```python
from build123d import *

# Parameters (mm, degrees)
REVOLUTION007_ANGLE     = 180
SKETCH064_W             = 14
SKETCH064_H             = 6
PAD026_DEPTH            = 10
SKETCH063_R             = 1.7
POCKET007_DEPTH         = 38.901
POCKET008_DEPTH         = 28.901
BODY015_PLACEMENT_ANGLE = 180


with BuildPart() as part:
    # Sketch062 → Revolution007 (revolve, symmetric)
    with BuildSketch(Plane.YZ) as revolution007_sk:
        with BuildLine():
            Line((32.9, 0), (32.9, 6.5))
            Line((32.9, 6.5), (29.4, 6.5))
            ThreePointArc((27.9, 8), (28.33934, 6.93934), (29.4, 6.5))
            Line((27.9, 8), (27.9, 11))
            ThreePointArc((29.4, 12.5), (28.33934, 12.06066), (27.9, 11))
            Line((29.4, 12.5), (32.9, 12.5))
            ThreePointArc((38.9, 6.5), (37.142641, 10.742641), (32.9, 12.5))
            Line((38.9, 6.5), (38.9, 0))
            Line((38.9, 0), (38.9, -6.5))
            ThreePointArc((32.9, -12.5), (37.142641, -10.742641), (38.9, -6.5))
            Line((32.9, -12.5), (29.4, -12.5))
            ThreePointArc((27.9, -11), (28.33934, -12.06066), (29.4, -12.5))
            Line((27.9, -11), (27.9, -8))
            ThreePointArc((29.4, -6.5), (28.33934, -6.93934), (27.9, -8))
            Line((29.4, -6.5), (32.9, -6.5))
            Line((32.9, -6.5), (32.9, 0))
        make_face()
    revolve(axis=Axis((0, 0, 0), (0, 0, 1)), revolution_arc=REVOLUTION007_ANGLE / 2)
    revolve(revolution007_sk.sketch, axis=Axis((0, 0, 0), (0, 0, -1)), revolution_arc=REVOLUTION007_ANGLE / 2)

    # Sketch064 (on Face18 of Revolution007) → Pad026 (new body)
    with BuildSketch(Plane(origin=(0, 0, 0), x_dir=(0, 0, -1), z_dir=(0, -1, 0))):
        with Locations((0, 39.4)):
            Rectangle(SKETCH064_W, SKETCH064_H)
        with Locations((0, -39.4)):
            Rectangle(SKETCH064_W, SKETCH064_H)
    extrude(amount=-PAD026_DEPTH)

    # Sketch063 (on Face18 of Revolution007) → Pocket007 (cut, through all)
    with BuildSketch(Plane(origin=(0, 0, 0), x_dir=(0, 0, -1), z_dir=(0, -1, 0))):
        with Locations((4, 39.4)):
            Circle(SKETCH063_R)
        with Locations((-4, 39.4)):
            Circle(SKETCH063_R)
        with Locations((-4, -39.4)):
            Circle(SKETCH063_R)
        with Locations((4, -39.4)):
            Circle(SKETCH063_R)
    extrude(amount=-POCKET007_DEPTH, mode=Mode.SUBTRACT)

    # Sketch065 (on Face22 of Pocket007) → Pocket008 (cut, through all)
    with BuildSketch(Plane.ZX.offset(10)):
        with BuildLine():
            Line((-4, 43.4), (4.000001, 43.4))
            ThreePointArc((4.000001, 35.4), (8, 39.4), (4.000001, 43.4))
            Line((-4, 35.4), (4.000001, 35.4))
            ThreePointArc((-4, 43.4), (-8, 39.4), (-4, 35.4))
        make_face()
        with BuildLine():
            Line((-4, -35.4), (4, -35.4))
            ThreePointArc((4, -43.4), (8, -39.4), (4, -35.4))
            Line((-4, -43.4), (4, -43.4))
            ThreePointArc((-4, -35.4), (-8, -39.4), (-4, -43.4))
        make_face()
    extrude(amount=POCKET008_DEPTH, mode=Mode.SUBTRACT)


with BuildPart() as part_1:
    # Body015 placement: moved
    add(part.part.moved(Location((0, 0, -0.5))).rotate(Axis((0, 0, -0.5), (1, 0, 0)), BODY015_PLACEMENT_ANGLE))


solid = part_1.part
```
Model file for the job. Use its own axes, mm. A direction names the side the tool comes from. Coordinates: 2 decimals unless noted, no trailing zeros. Loops run counter-clockwise (first coordinate to the right, second up) from the corner with the lowest first, then second, coordinate; pieces in that order, holes last. Notation, with made-up numbers: M 36.25,84.5 L 74.25,84.5 A3 ccw 74.25,89.5 Z; hole C -10.5,75.5 d8. An arc over 180 degrees is marked long. Use CSV: the item, a comma, the result in double quotes. Start each with the question number.
1. Tool access for faces 4 (the flat face through (39, -10, -1)), 5 (the cylindrical face through (41.086, -4.93, -4.721)), 6 (the flat face through (-2, -30, 6)), 7 (the flat face through (-39, -10, -1)), 8 (the flat face through (35, 0, -1)): list every direction of +Z, -Z, +X, -X, +Y, -Y with a clear straight run to the whole face (end or side of a thin tool).
2. Band-saw the part on B-B, the plane x = 0. List the corners of the cut face in (y, z), then the cut area to 3 significant figures.
3. Flat gauge pins, fed straight in: pin 1 (2 mm diameter, centred on x = -39.4, z = -4.5, fed in from +Y); pin 2 (8 mm diameter, centred on x = -21.5, z = -8.5, fed in from -Y); pin 3 (1 mm diameter, centred on y = -34.5, z = -5, fed in from +X); pin 4 (5.5 mm diameter, centred on x = 39.5, z = -3.5, fed in from -Y). Where does each tip first touch, or does it go through?
4. Two-plate mould, pull along X, no slides. Class faces 1 (the flat face through (-41, -5, 6.5)), 2 (the cylindrical face through (35.758, -12.339, 5.153)), 3 (the cylindrical face through (41.086, -4.93, 3.279)): pulls with the +X half, pulls with the -X half, needs draft (parallel to the pull), parting line crosses it, or undercut.
5. Band-saw the part on A-A, the plane z = -1.5. List the corners of the cut face in (x, y), then the cut area to 3 significant figures.
6. Probe probe 1 along Z at (x, y) = (-29.5, -13); probe 2 along X at (y, z) = (-5.75, -4.5); probe 3 along X at (y, z) = (-2.5, -4.5). List the from-to ranges inside material, lowest first. Write a range as [from, to].
7. Band-saw the part on C-C, the plane y = -6.5. Give the number of separate pieces and of enclosed holes in the cut face, then the cut area to 3 significant figures.
Entries:
1,face 4,"+X, -Y"
1,face 5,"+Y, -Y"
1,face 6,"+Y"
1,face 7,"-X, -Y"
1,face 8,"+Z, -Z, +X, -X, +Y"
2,outline,"M -38.9,-7 A6 ccw -32.9,-13 L -29.4,-13 A1.5 ccw -27.9,-11.5 L -27.9,-8.5 A1.5 ccw -29.4,-7 L -32.9,-7 L -32.9,6 L -29.4,6 A1.5 ccw -27.9,7.5 L -27.9,10.5 A1.5 ccw -29.4,12 L -32.9,12 A6 ccw -38.9,6 Z"
2,area,"193 mm2"
3,pin 1,"passes through"
3,pin 2,"stops at y = -34.66"
3,pin 3,"stops at x = 18.9"
3,pin 4,"stops at y = -10"
4,face 1,"needs draft"
4,face 2,"pulls with the +X half"
4,face 3,"undercut"
5,outline,"M -42.4,-10 L -35.4,-10 L -35.4,-16.13 A38.9 ccw 35.4,-16.13 L 35.4,-10 L 42.4,-10 L 42.4,0 L 32.9,0 A32.9 cw -32.9,0 L -42.4,0 Z"
5,area,"741 mm2"
6,probe 1,"z = [-13, -7], [6, 12]"
6,probe 2,"x = [-42.4, -41.1], [-37.7, -32.39], [32.39, 37.7], [41.1, 42.4]"
6,probe 3,"x = [-42.4, -41.1], [-37.7, -32.8], [32.8, 37.7], [41.1, 42.4]"
7,separate pieces,"2"
7,enclosed holes,"4"
7,area,"470 mm2"
